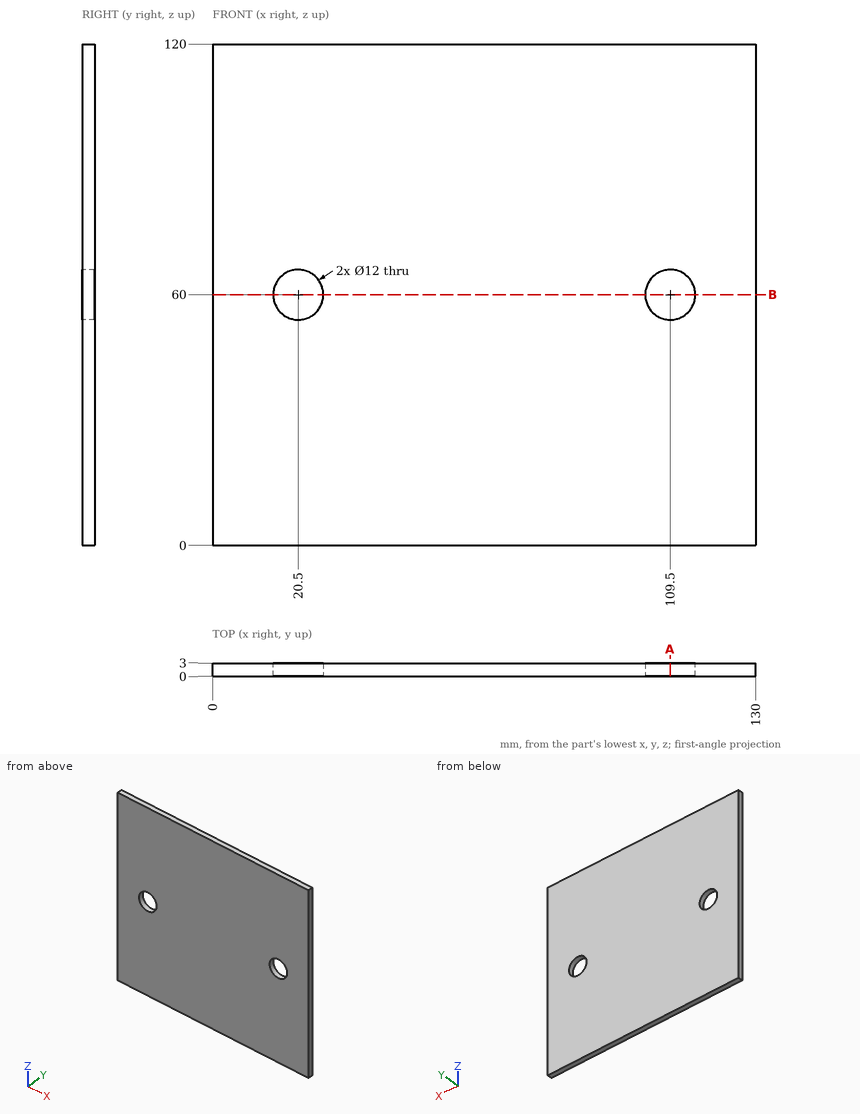
Study the drawing (mm; zero at the part's minimum x, y, z) and answer. Give positions to 0.01 mm unless a question says otherwise; leave off trailing zeros. Write each loop counter-clockwise with the first axis right and the second up, starting at its lowest first coordinate (ties: lowest second). Pieces come first, ordered by that corner, then holes. Notation, with made-up numbers: (70, 0) -> (106, 0) arc R30 cw to (106, 38) -> close; hole circle Ø11 at (-9.5, 13.25). An arc over 180 degrees is marked (long way). Write item = value, one per line. Start each with the question number.
1) Straight lines are drawn through the part: line 1 along Z through (x, y) = (109.5, 1.5); line 2 along X through (y, z) = (2.7, 63); line 3 along Z through (x, y) = (19.5, 1.3). For each, find the intervals that lie inside material, in ascending order.
2) The part is cut by section A-A, the plane x = 109.5. Determine the outline of the cut face in (y, z).
3) The part is cut by section B-B, the plane z = 60. Determine the outline of the cut face in (x, y), and give its area (3 significant figures).
Solutions:
q1.line_1 = 0 to 54, 66 to 120
q1.line_2 = 0 to 15.3, 25.7 to 104.3, 114.7 to 130
q1.line_3 = 0 to 54.08, 65.92 to 120
q2.outline = (0, 0) -> (3, 0) -> (3, 54) -> (0, 54) -> close; (0, 66) -> (3, 66) -> (3, 120) -> (0, 120) -> close
q3.outline = (0, 0) -> (14.5, 0) -> (14.5, 3) -> (0, 3) -> close; (26.5, 0) -> (103.5, 0) -> (103.5, 3) -> (26.5, 3) -> close; (115.5, 0) -> (130, 0) -> (130, 3) -> (115.5, 3) -> close
q3.area = 318 mm²
